Autodesk Inventor part; units mm, degrees
ref_plane "YZ Plane" through (0, 0, 0) normal (1, 0, 0) x (0, 1, 0)
ref_plane "XZ Plane" through (0, 0, 0) normal (0, 1, 0) x (-1, 0, 0)
ref_plane "XY Plane" through (0, 0, 0) normal (0, 0, 1) x (1, 0, 0)
sketch "Boceto1" plane through (0, 0, 0) normal (0, 1, 0) x (-1, 0, 0)
  arc A0 (-67.8307, -32) -> (67.8307, -32) centre (0, 0) ccw
  line L0 (0, -32) -> (-67.8307, -32)
  line L1 (0, -32) -> (67.8307, -32)
  dimension "d0" = 150
extrude "Extrusión1" add sketch "Boceto1" along normal blind 4
sketch "Boceto2" plane through (0, 4, 0) normal (0, 1, 0) x (1, 0, 0)
  line L0 (-67.8307, 32) -> (67.8307, 32)
  line L1 (0, 32) -> (0, 5)
  line L2 (0, 5) -> (-53, 5)
  line L3 (-53, 5) -> (-53, 82)
  line L4 (-53, 82) -> (53, 82)
  line L5 (53, 82) -> (53, 5)
  line L6 (53, 5) -> (0, 5)
  point P0 (0, 0)
  dimension "d4" = 27
  dimension "d5" = 53
  dimension "d6" = 77
  dimension "d7" = 106
extrude "Extrusión2" add sketch "Boceto2" along normal blind 11
sketch "Boceto3" plane through (0, 15, 0) normal (0, 1, 0) x (1, 0, 0)
  line L0 (53, 5) -> (53, 82)
  line L1 (53, 43.5) -> (53, 64.5)
  line L2 (40, 64.5) -> (-40, 64.5)
  line L3 (-53, 82) -> (-53, 5)
  line L4 (53, 82) -> (-53, 82)
  line L5 (0, 82) -> (40, 82)
  line L6 (40, 64.5) -> (40, 22.5)
  line L7 (-53, 5) -> (53, 5)
  line L8 (0, 82) -> (-40, 82)
  line L9 (-40, 64.5) -> (-40, 22.5)
  line L10 (53, 43.5) -> (53, 22.5)
  line L11 (40, 22.5) -> (-40, 22.5)
  point P0 (0, 0)
  dimension "d10" = 21
  dimension "d11" = 40
  dimension "d12" = 40
  dimension "d13" = 21
extrude "Extrusión3" cut sketch "Boceto3" against normal blind 7 contours L6 L11 L9 L2
sketch "Boceto4" plane through (40, 15, -22.5) normal (0, 0, -1) x (-1, 0, 0)
  line L0 (80, 0) -> (80, -7)
  line L1 (0, 0) -> (0, -7)
  line L2 (80, -7) -> (0, -7)
  line L3 (-13, 0) -> (-9, 0)
  line L4 (-9, 0) -> (0, 0)
  line L5 (0, 0) -> (0, -7)
  line L6 (0, -7) -> (-9, 0)
  line L7 (93, 0) -> (89, 0)
  line L8 (89, 0) -> (80, 0)
  line L9 (80, -7) -> (89, 0)
  point P0 (40, -15)
  dimension "d16" = 4
  dimension "d17" = 4
extrude "Extrusión4" cut sketch "Boceto4" along normal blind 55.5 and the other way blind 13.5
sketch "Boceto5" plane through (40, 8, -64.5) normal (1, 0, 0) x (0, 0, -1)
  line L0 (0, 7) -> (0, 0)
  line L1 (0, 0) -> (0, 7)
  line L2 (13.5, 7) -> (13.5, 0)
  line L3 (0, 7) -> (13.5, 7)
  line L4 (0, 0) -> (13.5, 0)
  line L5 (13.5, 7) -> (0, 0)
  line L6 (0, 0) -> (0, 7)
  line L7 (-42, 0) -> (0, 0)
  line L8 (-42, 7) -> (-42, 0)
  line L9 (-42, 0) -> (-42, 7)
  line L10 (-55.5, 7) -> (-55.5, 0)
  line L11 (-42, 7) -> (-55.5, 7)
  line L12 (-55.5, 0) -> (-42, 0)
  line L13 (-55.5, 7) -> (-42, 0)
  point P0 (-64.5, -8)
extrude "Extrusión5" cut sketch "Boceto5" against normal blind 80 contours L3 L5 L0 | L13 L11 L8
sketch "Boceto6" plane through (40, 8, -78) normal (1, 0, 0) x (0, 0, -1)
  line L0 (-69, 0) -> (-69, 7)
  line L1 (-69, 0) -> (-55.5, 0)
  line L2 (-69, 7) -> (-69, 0)
  line L3 (-69, 0) -> (-55.5, 0)
  line L4 (-69, 7) -> (0, 7)
  line L5 (-55.5, 0) -> (-69, 7)
  line L6 (0, 7) -> (0, 0)
  line L7 (0, 7) -> (0, 0)
  line L8 (-13.5, 0) -> (0, 7)
  line L9 (0, 0) -> (-13.5, 0)
  line L10 (0, 7) -> (-13.5, 0)
  point P0 (-78, -8)
extrude "Extrusión6" add sketch "Boceto6" along normal blind 10 and the other way blind 90
properties part number "Soporte_caja"
The listing builds one solid part. Answer for the finished solid, in the listing's coordinates (mm). A direction names the side the tool comes from. Give positions to 0.01 mm unless a question says otherwise; leave off trailing zeros. Write each loop counter-clockwise with the first axis right and the second up, starting at its lowest first coordinate (ties: lowest second). Pieces come first, ordered by that corner, then holes. Notation, with made-up numbers: (16.25, 52.5) - (36.25, 52.5) arc R23 ccw to (36.25, 74.5) - close; hole circle Ø10 at (-7, 29.25). An arc over 180 degrees is marked (long way). Use a Markdown table: item, result.
1. Section C-C on x = 22 is taken. Write down the section's boundary in (y, z), plus the area to 3 significant figures.
Values follow:
| item | result |
|---|---|
| outline | (0, -71.7) - (4, -71.7) - (4, -82) - (15, -82) - (15, -78) - (8, -64.5) - (8, -22.5) - (15, -9) - (15, -5) - (4, -5) - (4, -32) - (0, -32) - close |
| area | 617 mm² |
2. Each of these flat-tipped pins is pushed along its axis until it touches: P1, Ø6, axis at y = 5, z = -72, coming from the +X side; P2, Ø4, axis at y = 11, z = -47.5, coming from the -X side; P3, Ø1, axis at x = -12, z = -73, coming from the +Y side. Where does it stop, or does it pass through?
Values follow:
| item | result |
|---|---|
| P1 | stops at x = 53 |
| P2 | stops at x = -53 |
| P3 | stops at y = 12.67 |
3. Section B-B on z = -51 is taken. Write down the section's boundary in (x, y).
Values follow:
| item | result |
|---|---|
| outline | (-54.99, 0) - (54.99, 0) - (54.99, 4) - (53, 4) - (53, 15) - (49, 15) - (40, 8) - (-40, 8) - (-49, 15) - (-53, 15) - (-53, 4) - (-54.99, 4) - close |
4. Section D-D on y = 2 is taken. Write down the section's boundary in (x, z), plus the area to 3 significant figures.
Values follow:
| item | result |
|---|---|
| outline | (-67.83, -32) arc R75 ccw to (67.83, -32) - close |
| area | 4,190 mm² |
5. Section A-A on y = 9.75 is taken. Write down the section's boundary in (x, z) (3 decimals).
Values follow:
| item | result |
|---|---|
| outline | (-53, -82) - (53, -82) - (53, -5) - (-53, -5) - close; hole (-42.25, -67.875) - (42.25, -67.875) - (42.25, -19.125) - (-42.25, -19.125) - close |
6. For a pull along X with two mould halves and no side action, classify faces 1 (the flat face through (-1, 4, -19)), 2 (the flat face through (0.686, 11.549, -71.344)), 3 (the flat face through (-44.437, 11.451, -43.017)), 4 (the flat face through (-53, 9, -43)) as released by +X, released by -X, zero draft, split by the parting line, or undercut.
Values follow:
| item | result |
|---|---|
| face 1 | zero draft |
| face 2 | undercut |
| face 3 | undercut |
| face 4 | released by -X |
7. A tool of negligible diameter and unlimited length cuts with its end or side. For faces 5 (the flat face through (-0.686, 11.451, -15.845)), 6 (the flat face through (53, 9, -44)), 7 (the flat face through (-59, 4, -40)), 8 (the cylindrical face through (-1.19, 1.97, -74.99)), 9 (the flat face through (-1, 2, -32)), from which of +Z, -Z, +X, -X, +Y, -Y can it reach the whole face along a straight path? Write none if from no direction.
Values follow:
| item | result |
|---|---|
| face 5 | +Y |
| face 6 | +Z, -Z, +X, +Y |
| face 7 | +Z, -Z, -X, +Y |
| face 8 | -Z, -Y |
| face 9 | +Z, +X, -X, -Y |
8. Find the intervals of material crossed by probe 1 along Y at (x, z) = (-45, -9); probe 2 along Y at (x, z) = (10, -33.5); probe 3 along Z at (x, y) = (27, 9.5), in increasing order. Write a range as from..to.
Values follow:
| item | result |
|---|---|
| probe 1 | y = 4..15 |
| probe 2 | y = 0..8 |
| probe 3 | z = -82..-67.39, -19.61..-5 |
